Check sheet for the modelled part. Datum: model origin and axes. Units: mm. A direction names the side the tool comes from. Coordinates: 2 decimals unless noted, no trailing zeros. Write each loop counter-clockwise with the first axis right and the second up, starting at its lowest first coordinate (ties: lowest second). Pieces come first, ordered by that corner, then holes. Notation, with made-up numbers: (83, -13.5) - (93, -13.5) arc R17 ccw to (93, 3.5) - close; hole circle Ø6 at (86.5, 42). An arc over 180 degrees is marked (long way). Write each question's results on one line, items separated by ' | '.
from build123d import *

# Parameters (mm, degrees)
BASE_EXTRUDE_DEPTH = 12.7


with BuildPart() as part:
    # Sketch1 → Base-Extrude (new, symmetric)
    with BuildSketch(Plane.XY):
        with BuildLine():
            Line((-20.6375, 26.8351), (-20.6375, -6.9596))
            ThreePointArc((-20.6375, -6.9596), (-19.848914298, -8.863414298), (-17.9451, -9.652))
            Line((-17.9451, -9.652), (-50.8, -9.652))
            Line((-50.8, -9.652), (-50.8, -12.3444))
            Line((-50.8, -12.3444), (50.8, -12.3444))
            Line((50.8, -12.3444), (50.8, -9.652))
            Line((50.8, -9.652), (17.9451, -9.652))
            ThreePointArc((17.9451, -9.652), (19.848914298, -8.863414298), (20.6375, -6.9596))
            Line((20.6375, -6.9596), (20.6375, 26.8351))
            ThreePointArc((20.6375, 26.8351), (15.875, 31.5976), (11.1125, 26.8351))
            Line((11.1125, 26.8351), (11.1125, 25.80005))
            ThreePointArc((11.1125, 25.80005), (12.4587, 24.45385), (13.8049, 25.80005))
            Line((13.8049, 25.80005), (13.8049, 26.8351))
            ThreePointArc((13.8049, 26.8351), (15.875, 28.9052), (17.9451, 26.8351))
            Line((17.9451, 26.8351), (17.9451, -6.9596))
            Line((17.9451, -6.9596), (-17.9451, -6.9596))
            Line((-17.9451, -6.9596), (-17.9451, 26.8351))
            ThreePointArc((-17.9451, 26.8351), (-15.875, 28.9052), (-13.8049, 26.8351))
            Line((-13.8049, 26.8351), (-13.8049, 25.80005))
            ThreePointArc((-13.8049, 25.80005), (-12.4587, 24.45385), (-11.1125, 25.80005))
            Line((-11.1125, 25.80005), (-11.1125, 26.8351))
            ThreePointArc((-11.1125, 26.8351), (-15.875, 31.5976), (-20.6375, 26.8351))
        make_face()
    extrude(amount=BASE_EXTRUDE_DEPTH, both=True)


solid = part.part
1. Sectioned sample at B-B (z = -7.25). Record the cut outline in (x, y) (1 decimal), then the cut area to 3 significant figures.
Values follow:
outline: (-50.8, -12.3) - (50.8, -12.3) - (50.8, -9.7) - (17.9, -9.7) arc R2.7 ccw to (20.6, -7) - (20.6, 26.8) arc R4.8 ccw to (11.1, 26.8) - (11.1, 25.8) arc R1.3 ccw to (13.8, 25.8) - (13.8, 26.8) arc R2.1 cw to (17.9, 26.8) - (17.9, -7) - (-17.9, -7) - (-17.9, 26.8) arc R2.1 cw to (-13.8, 26.8) - (-13.8, 25.8) arc R1.3 ccw to (-11.1, 25.8) - (-11.1, 26.8) arc R4.8 ccw to (-20.6, 26.8) - (-20.6, -7) arc R2.7 ccw to (-17.9, -9.7) - (-50.8, -9.7) - close | area: 633 mm^2
2. Access from +Z, -Z, +X, -X, +Y, -Y to the whole of each face (thin tool, end or side, straight path). Record for faces 1 (the flat face through (-20.638, 10, 0)), 2 (the flat face through (20.638, 10, 0)), 3 (the cylindrical face through (12.429, 24.454, 0.178)).
Values follow:
face 1: +Z, -Z, -X, +Y | face 2: +Z, -Z, +X, +Y | face 3: +Z, -Z
3. Material ranges on L1, parallel to X at y = 5, z = -6.5; L2, parallel to Y at x = 10, z = -8.75; L3, parallel to Y at x = 43, z = -8, recorded low to high. Write a range as [from, to].
Values follow:
L1: x = [-20.64, -17.95], [17.95, 20.64] | L2: y = [-12.34, -6.96] | L3: y = [-12.34, -9.65]
4. Sectioned sample at A-A (y = 9). Record the cut outline in (x, z), then the cut area to 3 significant figures.
Values follow:
outline: (-20.64, -12.7) - (-17.95, -12.7) - (-17.95, 12.7) - (-20.64, 12.7) - close; (17.95, -12.7) - (20.64, -12.7) - (20.64, 12.7) - (17.95, 12.7) - close | area: 137 mm^2
5. Go/stop test with flat-tipped pins: pin 1 (12.5 mm diameter, centred on x = -30, z = -3.5, fed in from +Y); pin 2 (2 mm diameter, centred on y = 18.5, z = -2.5, fed in from -X); pin 3 (12 mm diameter, centred on y = -6, z = -9, fed in from -X); pin 4 (12.5 mm diameter, centred on y = 6.5, z = -6, fed in from +X). Record where each tip stops, or that it passes through.
Values follow:
pin 1: stops at y = -9.65 | pin 2: stops at x = -20.64 | pin 3: stops at x = -50.8 | pin 4: stops at x = 20.64
6. Sectioned sample at C-C (x = 1.5). Record the cut outline in (y, z).
Values follow:
outline: (-12.34, -12.7) - (-6.96, -12.7) - (-6.96, 12.7) - (-12.34, 12.7) - close
7. Sectioned sample at D-D (x = 30). Record the cut outline in (y, z).
Values follow:
outline: (-12.34, -12.7) - (-9.65, -12.7) - (-9.65, 12.7) - (-12.34, 12.7) - close
